from build123d import *

# Parameters (mm, degrees)
F0_R      = 1
F1_DEPTH  = 5.5
F3_DEPTH  = 25
F4_R      = 1
F5_DEPTH  = 11.001
F6_W      = 17.5
F6_H      = 8.5
F7_DEPTH  = 3
F8_R      = 1.25
F9_DEPTH  = 2
F10_R     = 1.5
F11_DEPTH = 1
F12_R     = 1.5
F13_DEPTH = 1
F15_DEPTH = 25


with BuildPart() as f1:
    # F0 (on Top) → F1 (new body, symmetric)
    with BuildSketch(Plane.XY):
        with BuildLine():
            Line((0, 56), (0, 0))
            Line((0, 0), (36.2259279858, 0))
            ThreePointArc((36.2259279858, 0), (38.7660402441, -1.4038077448), (38.9289329951, -4.3014468563))
            Line((38.9289329951, -4.3014468563), (28.817821884, -25.3014468563))
            ThreePointArc((28.817821884, -25.3014468563), (27.7110091299, -26.5401122582), (26.1148168747, -27))
            Line((26.1148168747, -27), (0, -27))
            Line((0, -27), (0, -33))
            Line((0, -33), (26.1148168747, -33))
            ThreePointArc((26.1148168747, -33), (30.9033936403, -31.6203367747), (34.2238319025, -27.904340569))
            Line((34.2238319025, -27.904340569), (43.9565924234, -7.690145641))
            ThreePointArc((43.9565924234, -7.690145641), (47.3319268627, -5.59281579), (50.7608266635, -7.6013777725))
            Line((50.7608266635, -7.6013777725), (84.9360533184, -64.560088864))
            ThreePointArc((84.9360533184, -64.560088864), (118.0198171676, -67.4369378944), (120.8966661979, -34.3531740452))
            Line((120.8966661979, -34.3531740452), (48.4995788875, 51.8338346577))
            ThreePointArc((48.4995788875, 51.8338346577), (44.4862343011, 54.9569066089), (39.5090393722, 56))
            Line((39.5090393722, 56), (29, 56))
            Line((29, 56), (29, 40))
            Line((29, 40), (14, 40))
            Line((14, 40), (14, 56))
            Line((14, 56), (0, 56))
        make_face()
        with Locations((34, 51)):
            Circle(F0_R, mode=Mode.SUBTRACT)
    extrude(amount=F1_DEPTH, both=True)

    # F2 (on face) → F3 (join)
    with BuildSketch(Plane(origin=(29, 0, 0), x_dir=(0, -1, 0), z_dir=(-1, 0, 0))):
        with BuildLine():
            ThreePointArc((-40, 5.5), (-45.5, 0), (-40, -5.5))
            Line((-40, -5.5), (-40, 5.5))
        make_face()
    extrude(amount=F3_DEPTH)

    # F4 (on face) → F5 (cut, through all)
    with BuildSketch(Plane.XY.offset(5.5)):
        with Locations((31, 20)):
            Circle(F4_R)
        with Locations((38, 20)):
            Circle(F4_R)
    extrude(amount=-F5_DEPTH, mode=Mode.SUBTRACT)

    # F6 (on face) → F7 (cut)
    with BuildSketch(Plane.XZ):
        with Locations((26.4759279858, 0)):
            Rectangle(F6_W, F6_H)
    extrude(amount=-F7_DEPTH, mode=Mode.SUBTRACT)

    # F8 (on face) → F9 (cut)
    with BuildSketch(Plane(origin=(53.9634146341, 45.3292682927, 0), x_dir=(-0.6431920864, 0.7657048648, 0), z_dir=(0.7657048648, 0.6431920864, 0))):
        with Locations((-31.5051259772, 0)):
            Circle(F8_R)
        with Locations((-7.5051259772, 0)):
            Circle(F8_R)
    extrude(amount=-F9_DEPTH, mode=Mode.SUBTRACT)

    # F10 (on face) → F11 (cut)
    with BuildSketch(Plane.XY.offset(5.5)):
        with Locations((7, 12.5)):
            Circle(F10_R)
        with Locations((31, 9)):
            Circle(F10_R)
    extrude(amount=-F11_DEPTH, mode=Mode.SUBTRACT)

    # F12 (on face) → F13 (cut)
    with BuildSketch(Plane(origin=(0, 0, -5.5), x_dir=(1, 0, 0), z_dir=(0, 0, -1))):
        with Locations((7, -12.5)):
            Circle(F12_R)
        with Locations((31, -9)):
            Circle(F12_R)
    extrude(amount=-F13_DEPTH, mode=Mode.SUBTRACT)

    # F14 (on face) → F15 (cut)
    with BuildSketch(Plane(origin=(0, 0, -5.5), x_dir=(1, 0, 0), z_dir=(0, 0, -1))):
        with BuildLine():
            Line((58.6916033415, 5.2701338496), (76.8614300391, -5.6317621689))
            Line((76.8614300391, -5.6317621689), (114.7710272796, 39.4987107366))
            ThreePointArc((114.7710272796, 39.4987107366), (113.0903982462, 61.1263473001), (91.4355349705, 59.8433532312))
            Line((91.4355349705, 59.8433532312), (58.6916033415, 5.2701338496))
        make_face()
    extrude(amount=-F15_DEPTH, mode=Mode.SUBTRACT)


solid = f1.part
Source: CAD feature listing. Evaluate the final solid. Frame: model axes, mm. A direction names the side the tool comes from. Coordinates: 2 decimals unless noted, no trailing zeros. Loops run counter-clockwise (first coordinate to the right, second up) from the corner with the lowest first, then second, coordinate; pieces in that order, holes last. Notation, with made-up numbers: M 63,16 L 116,16 A28 cw 116,54 Z; hole C 37.25,-6 d11. An arc over 180 degrees is marked long. Answer in a Markdown table with one row per item.
Q1. Section A-A on x = 12. Return the cut outline in (y, z).
Answers below:
| item | result |
|---|---|
| outline | M -33,-5.5 L -27,-5.5 L -27,5.5 L -33,5.5 Z; M 0,-5.5 L 56,-5.5 L 56,5.5 L 0,5.5 Z |
Q2. First-contact query: pin 1 (1 mm diameter, centred on y = -60, z = -4.5, fed in from +X); pin 2 (1 mm diameter, centred on y = -5, z = -3.5, fed in from -X); pin 3 (1.5 mm diameter, centred on x = 7, y = 13, fed in from +Z). Flat tips, straight axial feed; report the tip coordinate or a pass-through.
Answers below:
| item | result |
|---|---|
| pin 1 | stops at x = 124.14 |
| pin 2 | stops at x = 38.35 |
| pin 3 | stops at z = 4.5 |
Q3. Ray query, probe 1 along Y at (x, z) = (7, -4.9); probe 2 along Y at (x, z) = (10.5, 4.25); probe 3 along X at (y, z) = (50.5, -3.75). Return the intervals inside material, ascending. Write a range as from..to.
Answers below:
| item | result |
|---|---|
| probe 1 | y = -33..-27, 0..11, 14..56 |
| probe 2 | y = -33..-27, 0..56 |
| probe 3 | x = 0..14, 29..33.13, 34.87..49.62 |
Q4. Draft query along Y for faces 4 (the flat face through (26, 1, -4.25)), 5 (the cylindrical face through (30.84, -31.66, 0.08)), 6 (the flat face through (0, 28, 0)). Return one class per face: pulls with the +Y half, pulls with the -Y half, needs draft (parallel to the pull), parting line crosses it, or undercut.
Answers below:
| item | result |
|---|---|
| face 4 | undercut |
| face 5 | pulls with the -Y half |
| face 6 | needs draft |
Q5. Set-up query: faces 1 (the cylindrical face through (29.5, 8.93, -5.01)), 2 (the cylindrical face through (21.6, 45.5, 0.1)), 3 (the flat face through (13, -27, 0)). Return all of +Z, -Z, +X, -X, +Y, -Y with unobstructed straight access to the full face (end or side cutting, diameter ignored); none if empty.
Answers below:
| item | result |
|---|---|
| face 1 | -Z |
| face 2 | +Y |
| face 3 | +Z, -Z, -X |
Q6. Section C-C on x = 68.5. Return the cut outline in (y, z), plus the area to 3 significant figures.
Answers below:
| item | result |
|---|---|
| outline | M -37.17,-5.5 L -21.62,-5.5 L -21.62,5.5 L -37.17,5.5 Z; M 0.61,-5.5 L 28.02,-5.5 L 28.02,5.5 L 0.61,5.5 Z |
| area | 473 mm^2 |
Q7. Section D-D on y = -11. Return the cut outline in (x, z).
Answers below:
| item | result |
|---|---|
| outline | M 35.7,-5.5 L 42.36,-5.5 L 42.36,5.5 L 35.7,5.5 Z; M 52.8,-5.5 L 62.13,-5.5 L 62.13,5.5 L 52.8,5.5 Z; M 90.83,-5.5 L 101.28,-5.5 L 101.28,5.5 L 90.83,5.5 Z |
Q8. Section B-B on y = 9. Return the cut outline in (x, z), plus the area to 3 significant figures.
Answers below:
| item | result |
|---|---|
| outline | M 0,-5.5 L 29.5,-5.5 L 29.5,-4.5 L 32.5,-4.5 L 32.5,-5.5 L 84.48,-5.5 L 84.48,5.5 L 32.5,5.5 L 32.5,4.5 L 29.5,4.5 L 29.5,5.5 L 0,5.5 Z |
| area | 923 mm^2 |
